Part model, mm, in its own coordinate system. A direction names the side the tool comes from. Give positions to 0.01 mm unless a question says otherwise; leave off trailing zeros. Write each loop counter-clockwise with the first axis right and the second up, starting at its lowest first coordinate (ties: lowest second). Pieces come first, ordered by that corner, then holes.
from build123d import *

# Parameters (mm, degrees)
ESQUISSE1_R             = 2.5
BOSS_EXTRU_1_DEPTH      = 8
ESQUISSE2_R             = 3.15
BOSS_EXTRU_2_DEPTH      = 1.5
CHANFREIN1_SIZE         = 1.5
ENL_V_MAT_EXTRU_1_DEPTH = 1.5


with BuildPart() as part:
    # Esquisse1 → Boss.-Extru.1 (new body)
    with BuildSketch(Plane.XY):
        Circle(ESQUISSE1_R)
    extrude(amount=BOSS_EXTRU_1_DEPTH)

    # Esquisse2 → Boss.-Extru.2 (add)
    with BuildSketch(Plane.XY.offset(8)):
        Circle(ESQUISSE2_R)
    extrude(amount=BOSS_EXTRU_2_DEPTH)

    # Chanfrein1
    # the kernel refuses this chamfer: 1.5 mm, written as the material it takes off along each edge
    with BuildSketch(Plane(origin=(0, 0, 8), x_dir=(1, 0, 0), z_dir=(0, -1, 0))) as chanfrein1_piece_1_section:
        Polygon((3.15, CHANFREIN1_SIZE), (3.15 - CHANFREIN1_SIZE, 0), (3.15, 0), align=None)
    chanfrein1_piece_1 = revolve(axis=Axis((0, 0, 8), (0, 0, 1)), mode=Mode.PRIVATE)
    chanfrein1_piece_1 = chanfrein1_piece_1 - Plane(origin=(0, 0, 9.178723354), x_dir=(1, 0, 0), z_dir=(0, 0, -1)) * Cylinder(2.5, 13, mode=Mode.PRIVATE)
    add(chanfrein1_piece_1, mode=Mode.SUBTRACT)

    # Esquisse3 → Enlèv. mat.-Extru.1 (cut)
    with BuildSketch(Plane.XY.offset(9.5)):
        Polygon((-0.6, 2.1), (0.6, 2.1), (0.6, 0.6), (2.1, 0.6), (2.1, -0.6), (0.6, -0.6), (0.6, -2.1), (-0.6, -2.1), (-0.6, -0.6), (-2.1, -0.6), (-2.1, 0.6), (-0.6, 0.6), align=None)
    extrude(amount=-ENL_V_MAT_EXTRU_1_DEPTH, mode=Mode.SUBTRACT)


solid = part.part
1) Saw through at A-A (x = 0). Write the cut outline in (y, z), and give its area (3 significant figures).
Check result:
outline: (-3.15, 9.5) - (-2.5, 8.85) - (-2.5, 0) - (2.5, 0) - (2.5, 8.85) - (3.15, 9.5) - (2.1, 9.5) - (2.1, 8) - (-2.1, 8) - (-2.1, 9.5) - close
area: 41.6 mm2
2) Drill centre lines: L1, parallel to Y at x = 0, z = 5.5; L2, parallel to Z at x = -1, y = 0.25; L3, parallel to Y at x = 0.25, z = 8.5. Where is each one in solid material? Low to high.
Check result:
L1: y = -2.5 to 2.5
L2: z = 0 to 8
L3: y = -2.49 to -2.1, 2.1 to 2.49
3) 3-axis set-ups, long thin cutter, end or side, ignore diameter. For faces 4 (the flat face through (1, -1, 9.5)), 5 (the flat face through (-0.6, -1, 9)): which of +Z, -Z, +X, -X, +Y, -Y reach the whole face in a straight line?
Check result:
face 4: +Z, +X, -X, +Y, -Y
face 5: +Z
4) Saw through at C-C (z = 5.75). Write the cut outline in (x, y).
Check result:
outline: circle Ø5 at (0, 0)
5) Flat gauge pins, fed straight in: P1, Ø1.2, axis at y = 1.5, z = 9, coming from the -X side; P2, Ø0.8, axis at x = 1.5, z = 9, coming from the -Y side; P3, Ø0.8, axis at y = 1.5, z = 8.5, coming from the +X side (3 decimals). Where does each tip first touch, or does it go through?
Check result:
P1: stops at x = -2.93
P2: stops at y = -2.7
P3: stops at x = 2.245
6) Mould opens along Y. For faces 1 (the flat face through (0, 0, 0)), 2 (the flat face through (0, 2.1, 9)), 3 (the flat face through (0.6, -1, 9)) say: +Y half, -Y half, draft (parallel to the pull), parting line (faces both ways), or undercut.
Check result:
face 1: draft
face 2: undercut
face 3: undercut
